Read the model definition and answer for the solid it produces. Units are mm, in the model's axes. A direction names the side the tool comes from. Give positions to 0.01 mm unless a question says otherwise; leave off trailing zeros. Write each loop counter-clockwise with the first axis right and the second up, starting at its lowest first coordinate (ties: lowest second). Pieces come first, ordered by that corner, then holes. Notation, with made-up numbers: M 12,-30.5 L 22,-30.5 A30 cw 22,3.5 Z; hole C 63.5,-7 d3. An arc over 180 degrees is marked long. Put each result on its own line as item: value.
from build123d import *

# Parameters (mm, degrees)
SKETCH_1_R          = 5
SKETCH_1_W          = 70
SKETCH_1_H          = 6
EXTRUDE_1_DEPTH     = 2
SKETCH_1_3_R        = 2
CUT_EXTRUDE_1_DEPTH = 76.266194271
FILLET_1_R          = 3


with BuildPart() as part:
    # 草图1 → 凸台-拉伸1 (new body)
    with BuildSketch(Plane(origin=(0, 0, 0), x_dir=(0, 0, -1), z_dir=(1, 0, 0))):
        with Locations((70, -1)):
            Circle(SKETCH_1_R)
        with Locations((0, -1)):
            Circle(SKETCH_1_R)
        with Locations((35, -3)):
            Rectangle(SKETCH_1_W, SKETCH_1_H)
    extrude(amount=EXTRUDE_1_DEPTH)

    # 草图1<3> → 切除-拉伸1 (cut, through all)
    with BuildSketch(Plane(origin=(0, 0, 0), x_dir=(0, 0, -1), z_dir=(1, 0, 0))):
        with Locations((70, -1)):
            Circle(SKETCH_1_3_R)
        with Locations((0, -1)):
            Circle(SKETCH_1_3_R)
    extrude(amount=CUT_EXTRUDE_1_DEPTH, mode=Mode.SUBTRACT)

    # 圆角1
    fillet_1_edges = [part.edges().sort_by_distance(p)[0] for p in [
        (1, 0, -65.101020514),
        (1, 0, -4.898979486),
    ]]
    fillet(fillet_1_edges, radius=FILLET_1_R)


solid = part.part
(1) Section C-C on y = 2.5 is taken. Determine the outline of the cut face in (x, z).
Result:
outline: M 0,-73.57 L 2,-73.57 L 2,-66.43 L 0,-66.43 Z; M 0,-3.57 L 2,-3.57 L 2,3.57 L 0,3.57 Z
(2) Which of the six approach directions +Z, -Z, +X, -X, +Y, -Y give full straight-line access (tool end or side, diameter ignored) to faces 1 (the face through (0.986, -0.399, -1.908)), 2 (the face through (1, 0, -35))?
Result:
face 1: +X, -X
face 2: +X, -X, +Y
(3) Straight lines are drawn through the part: line 1 along Z through (x, y) = (1.5, -1); line 2 along Z through (x, y) = (1.5, 0.5); line 3 along Z through (x, y) = (0.1, 0.25). For each, find the intervals that lie inside material, in ascending order. Write a range as from..to.
Result:
line 1: z = -75..-72, -68..-2, 2..5
line 2: z = -74.77..-71.32, -68.68..-64.73, -5.27..-1.32, 1.32..4.77
line 3: z = -74.84..-71.56, -68.44..-64.27, -5.73..-1.56, 1.56..4.84
(4) Section A-A on y = -1 is taken. Determine the outline of the cut face in (x, z).
Result:
outline: M 0,-75 L 2,-75 L 2,-72 L 0,-72 Z; M 0,-68 L 2,-68 L 2,-2 L 0,-2 Z; M 0,2 L 2,2 L 2,5 L 0,5 Z
(5) For a pull along Y with two mould halves and no side action, classify faces 3 (the face through (1.01, 0.39, -64.55)), 4 (the face through (1, -6, -35)), 5 (the face through (0.986, -0.399, -71.908)) as +Y half, -Y half, draft (parallel to the pull), parting line (faces both ways), or undercut.
Result:
face 3: +Y half
face 4: -Y half
face 5: undercut
(6) Section B-B on x = 0.3 is taken. Determine the outline of the cut face in (y, z), and give its area (3 significant figures).
Result:
outline: M -6,-70 A5 ccw long 1.5,-65.67 A3 cw 0,-63.07 L 0,-6.93 A3 cw 1.5,-4.33 A5 ccw long -6,0 Z; hole C -1,-70 d4; hole C -1,0 d4
area: 504 mm²
(7) Section D-D on z = -27.5 is taken. Determine the outline of the cut face in (x, y), and give its area (3 significant figures).
Result:
outline: M 0,-6 L 2,-6 L 2,0 L 0,0 Z
area: 12.0 mm²
